Verification items for the finished model (mm, model axes). A direction names the side the tool comes from. Give positions to 0.01 mm unless a question says otherwise; leave off trailing zeros. Loops run counter-clockwise (first coordinate to the right, second up) from the corner with the lowest first, then second, coordinate; pieces in that order, holes last. Notation, with made-up numbers: (-20.75, 81.5) - (-9.75, 81.5) arc R18 cw to (-9.75, 96.5) - close; hole circle Ø1 at (23.25, 2.25). An arc over 180 degrees is marked (long way). One line per question, with ' | ' between items. Start each with the question number.
1. Tool access check on faces 4 (the face through (-18.764, 1.134, 3.531)), 5 (the face through (-16.17, 28.75, 0.39)), 6 (the face through (-16.167, 28.753, 6.599)). Record the directions out of +Z, -Z, +X, -X, +Y, -Y that give a thin tool (end or side, any length) a straight path to the whole face; none if there is none.
2. Section check B-B, the plane z = 2.5. Enter the section's corners in (x, y) (1 decimal).
3. Depth check by flat-ended pin: pin 1 Ø3 at (y, z) = (20, 3.5) entering from +X; pin 2 Ø4 at (y, z) = (-16.5, 1.5) entering from +X; pin 3 Ø1 at (x, y) = (22, 1) entering from -Z; pin 4 Ø1.6 at (x, z) = (31.5, 3.5) entering from +Y. Enter the tip coordinate at first touch or a pass-through.
4. Section check C-C, the plane x = 40.5. Enter the section's corners in (y, z) (3 decimals).
5. Thickness scan on line 1 along Y through (x, z) = (-9, 1.75); line 2 along Y through (x, z) = (-21, 0.5); line 3 along Y through (x, z) = (-15, 1.5). Record the ranges inside material, lowest first. Write a range as from..to.
6. Mould release check, pull along Y, two halves, no side actions. Record for faces 1 (the face through (47.587, -2.912, 0.132)), 2 (the face through (39.253, -22.945, 3.454)), 3 (the face through (-15.09, 8.79, 3.45)): +Y half, -Y half, draft (parallel to the pull), parting line (faces both ways), or undercut.
7. Section check A-A, the plane y = -32. Enter the section's corners in (x, z) (3 decimals), then the cut area to 3 significant figures.
from build123d import *

# Parameters (mm, degrees)
F1_DEPTH = 6.985
F2_R     = 5.08
F3_SIZE  = 0.762


with BuildPart() as f1:
    # F0 (on Top) → F1 (new body)
    with BuildSketch(Plane.XY):
        with BuildLine():
            ThreePointArc((-7.41045, 12.8352759069), (-3.8359311856, 14.3158900788), (0, 14.8209))
            Line((0, 14.8209), (0, 17.4625))
            ThreePointArc((0, 17.4625), (-4.5196275751, 16.8674797416), (-8.73125, 15.1229686136))
            Line((-8.73125, 15.1229686136), (-7.41045, 12.8352759069))
        make_face()
        with BuildLine():
            Line((0, 17.4625), (0, 14.8209))
            ThreePointArc((0, 14.8209), (3.8359311856, 14.3158900788), (7.41045, 12.8352759069))
            Line((7.41045, 12.8352759069), (8.73125, 15.1229686136))
            ThreePointArc((8.73125, 15.1229686136), (4.5196275751, 16.8674797416), (0, 17.4625))
        make_face()
        with BuildLine():
            ThreePointArc((14.8209, 0), (14.3158900788, -3.8359311856), (12.8352759069, -7.41045))
            Line((12.8352759069, -7.41045), (15.1229686136, -8.73125))
            ThreePointArc((15.1229686136, -8.73125), (16.8674797416, -4.5196275751), (17.4625, 0))
            Line((17.4625, 0), (14.8209, 0))
        make_face()
        with BuildLine():
            Line((15.1229686136, -8.73125), (12.8352759069, -7.41045))
            ThreePointArc((12.8352759069, -7.41045), (10.4799588933, -10.4799588933), (7.41045, -12.8352759069))
            Line((7.41045, -12.8352759069), (8.73125, -15.1229686136))
            ThreePointArc((8.73125, -15.1229686136), (12.3478521665, -12.3478521665), (15.1229686136, -8.73125))
        make_face()
        with BuildLine():
            ThreePointArc((-7.41045, -12.8352759069), (-10.4799588933, -10.4799588933), (-12.8352759069, -7.41045))
            Line((-12.8352759069, -7.41045), (-15.1229686136, -8.73125))
            ThreePointArc((-15.1229686136, -8.73125), (-12.3478521665, -12.3478521665), (-8.73125, -15.1229686136))
            Line((-8.73125, -15.1229686136), (-7.41045, -12.8352759069))
        make_face()
        with BuildLine():
            Line((-15.1229686136, -8.73125), (-12.8352759069, -7.41045))
            ThreePointArc((-12.8352759069, -7.41045), (-14.3158900788, -3.8359311856), (-14.8209, 0))
            Line((-14.8209, 0), (-17.4625, 0))
            ThreePointArc((-17.4625, 0), (-16.8674797416, -4.5196275751), (-15.1229686136, -8.73125))
        make_face()
        with BuildLine():
            ThreePointArc((-8.73125, 15.1229686136), (-4.5196275751, 16.8674797416), (0, 17.4625))
            Line((0, 17.4625), (0, 19.4691))
            ThreePointArc((0, 19.4691), (-11.0109, 30.48), (0, 41.4909))
            Line((0, 41.4909), (0, 45.466))
            Line((0, 45.466), (-26.249807339, 45.466))
            Line((-26.249807339, 45.466), (-8.73125, 15.1229686136))
        make_face()
        with BuildLine():
            Line((0, 19.4691), (0, 17.4625))
            ThreePointArc((0, 17.4625), (4.5196275751, 16.8674797416), (8.73125, 15.1229686136))
            Line((8.73125, 15.1229686136), (26.249807339, 45.466))
            Line((26.249807339, 45.466), (0, 45.466))
            Line((0, 45.466), (0, 41.4909))
            ThreePointArc((0, 41.4909), (7.785882057, 38.265882057), (11.0109, 30.48))
            ThreePointArc((11.0109, 30.48), (7.785882057, 22.694117943), (0, 19.4691))
        make_face()
        with BuildLine():
            Line((8.73125, 15.1229686136), (7.41045, 12.8352759069))
            ThreePointArc((7.41045, 12.8352759069), (12.8352759069, 7.41045), (14.8209, 0))
            Line((14.8209, 0), (17.4625, 0))
            ThreePointArc((17.4625, 0), (15.1229686136, 8.73125), (8.73125, 15.1229686136))
        make_face()
        with BuildLine():
            ThreePointArc((-14.8209, 0), (-12.8352759069, 7.41045), (-7.41045, 12.8352759069))
            Line((-7.41045, 12.8352759069), (-8.73125, 15.1229686136))
            ThreePointArc((-8.73125, 15.1229686136), (-15.1229686136, 8.73125), (-17.4625, 0))
            Line((-17.4625, 0), (-14.8209, 0))
        make_face()
        with BuildLine():
            ThreePointArc((17.4625, 0), (16.8674797416, -4.5196275751), (15.1229686136, -8.73125))
            Line((15.1229686136, -8.73125), (16.8607351888, -9.73455))
            ThreePointArc((16.8607351888, -9.73455), (29.2462849311, -4.6042873193), (37.4073543073, -15.24))
            ThreePointArc((37.4073543073, -15.24), (37.032166988, -18.0898306237), (35.9321734259, -20.74545))
            Line((35.9321734259, -20.74545), (39.3747110085, -22.733))
            Line((39.3747110085, -22.733), (52.499614678, 0))
            Line((52.499614678, 0), (17.4625, 0))
        make_face()
        with BuildLine():
            Line((16.8607351888, -9.73455), (15.1229686136, -8.73125))
            ThreePointArc((15.1229686136, -8.73125), (12.3478521665, -12.3478521665), (8.73125, -15.1229686136))
            Line((8.73125, -15.1229686136), (26.249807339, -45.466))
            Line((26.249807339, -45.466), (39.3747110085, -22.733))
            Line((39.3747110085, -22.733), (35.9321734259, -20.74545))
            ThreePointArc((35.9321734259, -20.74545), (20.8910043073, -24.7757191185), (16.8607351888, -9.73455))
        make_face()
        with BuildLine():
            Line((8.73125, -15.1229686136), (7.41045, -12.8352759069))
            ThreePointArc((7.41045, -12.8352759069), (0, -14.8209), (-7.41045, -12.8352759069))
            Line((-7.41045, -12.8352759069), (-8.73125, -15.1229686136))
            ThreePointArc((-8.73125, -15.1229686136), (0, -17.4625), (8.73125, -15.1229686136))
        make_face()
        with BuildLine():
            ThreePointArc((-8.73125, -15.1229686136), (-12.3478521665, -12.3478521665), (-15.1229686136, -8.73125))
            Line((-15.1229686136, -8.73125), (-16.8607351888, -9.73455))
            ThreePointArc((-16.8607351888, -9.73455), (-15.7607416267, -12.3901693763), (-15.3855543073, -15.24))
            ThreePointArc((-15.3855543073, -15.24), (-23.5466236836, -25.8757126807), (-35.9321734259, -20.74545))
            Line((-35.9321734259, -20.74545), (-39.3747110085, -22.733))
            Line((-39.3747110085, -22.733), (-26.249807339, -45.466))
            Line((-26.249807339, -45.466), (-8.73125, -15.1229686136))
        make_face()
        with BuildLine():
            Line((-16.8607351888, -9.73455), (-15.1229686136, -8.73125))
            ThreePointArc((-15.1229686136, -8.73125), (-16.8674797416, -4.5196275751), (-17.4625, 0))
            Line((-17.4625, 0), (-52.499614678, 0))
            Line((-52.499614678, 0), (-39.3747110085, -22.733))
            Line((-39.3747110085, -22.733), (-35.9321734259, -20.74545))
            ThreePointArc((-35.9321734259, -20.74545), (-31.9019043073, -5.7042808815), (-16.8607351888, -9.73455))
        make_face()
        with BuildLine():
            ThreePointArc((-9.5357191185, -5.50545), (-9.5357191185, 5.50545), (0, 11.0109))
            Line((0, 11.0109), (0, 14.8209))
            ThreePointArc((0, 14.8209), (-3.8359311856, 14.3158900788), (-7.41045, 12.8352759069))
            ThreePointArc((-7.41045, 12.8352759069), (-12.8352759069, 7.41045), (-14.8209, 0))
            ThreePointArc((-14.8209, 0), (-14.3158900788, -3.8359311856), (-12.8352759069, -7.41045))
            Line((-12.8352759069, -7.41045), (-9.5357191185, -5.50545))
        make_face()
        with BuildLine():
            ThreePointArc((0, 11.0109), (7.785882057, 7.785882057), (11.0109, 0))
            ThreePointArc((11.0109, 0), (10.6357126807, -2.8498306237), (9.5357191185, -5.50545))
            Line((9.5357191185, -5.50545), (12.8352759069, -7.41045))
            ThreePointArc((12.8352759069, -7.41045), (14.3158900788, -3.8359311856), (14.8209, 0))
            ThreePointArc((14.8209, 0), (12.8352759069, 7.41045), (7.41045, 12.8352759069))
            ThreePointArc((7.41045, 12.8352759069), (3.8359311856, 14.3158900788), (0, 14.8209))
            Line((0, 14.8209), (0, 11.0109))
        make_face()
        with BuildLine():
            Line((12.8352759069, -7.41045), (9.5357191185, -5.50545))
            ThreePointArc((9.5357191185, -5.50545), (0, -11.0109), (-9.5357191185, -5.50545))
            Line((-9.5357191185, -5.50545), (-12.8352759069, -7.41045))
            ThreePointArc((-12.8352759069, -7.41045), (-10.4799588933, -10.4799588933), (-7.41045, -12.8352759069))
            ThreePointArc((-7.41045, -12.8352759069), (0, -14.8209), (7.41045, -12.8352759069))
            ThreePointArc((7.41045, -12.8352759069), (10.4799588933, -10.4799588933), (12.8352759069, -7.41045))
        make_face()
    extrude(amount=F1_DEPTH)

    # F2
    f2_edges = [f1.edges().sort_by_distance(p)[0] for p in [
        (8.73125, -15.122969, 3.4925),
        (26.249807, -45.466, 3.4925),
        (52.499615, 0, 3.4925),
        (17.4625, 0, 3.4925),
        (8.73125, 15.122969, 3.4925),
        (26.249807, 45.466, 3.4925),
        (-26.249807, 45.466, 3.4925),
        (-8.73125, 15.122969, 3.4925),
        (-17.4625, 0, 3.4925),
        (-52.499615, 0, 3.4925),
        (-26.249807, -45.466, 3.4925),
        (-8.73125, -15.122969, 3.4925),
    ]]
    fillet(f2_edges, radius=F2_R)

    # F3
    f3_edges = [f1.edges().sort_by_distance(p)[0] for p in [
        (-32.831722, 0, 6.985),
        (-16.415861, 28.433106, 6.985),
        (32.831722, 0, 6.985),
        (16.415861, 28.433106, 6.985),
        (0, 45.466, 6.985),
        (-39.374711, -22.733, 6.985),
        (39.374711, -22.733, 6.985),
        (16.415861, -28.433106, 6.985),
        (-16.415861, -28.433106, 6.985),
        (-16.415861, -28.433106, 0),
        (-32.831722, 0, 0),
        (-16.415861, 28.433106, 0),
        (16.415861, 28.433106, 0),
        (32.831722, 0, 0),
        (16.415861, -28.433106, 0),
        (39.374711, -22.733, 0),
        (0, 45.466, 0),
        (-39.374711, -22.733, 0),
        (8.444714, -16.834073, 0),
        (26.249807, -40.386, 0),
        (0, -17.4625, 0),
        (-8.444714, -16.834073, 0),
        (48.100206, -2.54, 0),
        (-26.249807, -40.386, 0),
        (18.801092, 1.1037, 0),
        (15.122969, 8.73125, 0),
        (-48.100206, -2.54, 0),
        (10.356378, 15.730373, 0),
        (-18.801092, 1.1037, 0),
        (21.850398, 42.926, 0),
        (-15.122969, 8.73125, 0),
        (-10.356378, 15.730373, 0),
        (-21.850398, 42.926, 0),
        (8.444714, -16.834073, 6.985),
        (26.249807, -40.386, 6.985),
        (0, -17.4625, 6.985),
        (-8.444714, -16.834073, 6.985),
        (48.100206, -2.54, 6.985),
        (-26.249807, -40.386, 6.985),
        (18.801092, 1.1037, 6.985),
        (15.122969, 8.73125, 6.985),
        (-48.100206, -2.54, 6.985),
        (10.356378, 15.730373, 6.985),
        (-18.801092, 1.1037, 6.985),
        (21.850398, 42.926, 6.985),
        (-15.122969, 8.73125, 6.985),
        (-10.356378, 15.730373, 6.985),
        (-21.850398, 42.926, 6.985),
    ]]
    chamfer(f3_edges, length=F3_SIZE)


solid = f1.part
Results list:
1) face 4: +Z, -Z, -X | face 5: -Z, -X | face 6: +Z, -X
2) outline: (-48.1, -7.6) - (-30.6, -37.8) arc R5.1 ccw to (-21.9, -37.8) - (-11, -19) arc R5.1 cw to (-5.1, -16.7) arc R17.5 ccw to (5.1, -16.7) arc R5.1 cw to (11, -19) - (21.9, -37.8) arc R5.1 ccw to (30.6, -37.8) - (48.1, -7.6) arc R5.1 ccw to (43.7, 0) - (22, 0) arc R5.1 cw to (17, 3.9) arc R17.5 ccw to (11.9, 12.8) arc R5.1 cw to (11, 19) - (21.9, 37.8) arc R5.1 ccw to (17.5, 45.5) - (-17.5, 45.5) arc R5.1 ccw to (-21.9, 37.8) - (-11, 19) arc R5.1 cw to (-11.9, 12.8) arc R17.5 ccw to (-17, 3.9) arc R5.1 cw to (-22, 0) - (-43.7, 0) arc R5.1 ccw to start; hole circle Ø22 at (-26.4, -15.2); hole circle Ø22 at (0, 0); hole circle Ø22 at (0, 30.5); hole circle Ø22 at (26.4, -15.2)
3) pin 1: x = 12.41 | pin 2: x = 44.13 | pin 3: through | pin 4: y = 0
4) outline: (-20.784, 0.762) - (-19.26, 0) - (-0.762, 0) - (0, 0.762) - (0, 6.223) - (-0.762, 6.985) - (-19.26, 6.985) - (-20.784, 6.223) - close
5) line 1: -17.09..-6.34, 6.34..24.14, 36.82..45.47 | line 2: -35.85..-24.84, -5.64..-0.17, 36.9..43.64 | line 3: -25.98..8.94, 25.98..45.47
6) face 1: parting line | face 2: -Y half | face 3: undercut
7) outline: (-34.024, 0.762) - (-33.145, 0) - (-19.355, 0) - (-18.475, 0.762) - (-18.475, 6.223) - (-19.355, 6.985) - (-33.145, 6.985) - (-34.024, 6.223) - close; (18.475, 0.762) - (19.355, 0) - (33.145, 0) - (34.024, 0.762) - (34.024, 6.223) - (33.145, 6.985) - (19.355, 6.985) - (18.475, 6.223) - close | area: 215 mm²
